from build123d import *

# Parameters (mm, degrees)
SKETCH1_R           = 1.8
BOSS_EXTRUDE1_DEPTH = 2
SKETCH2_W           = 12
SKETCH2_H           = 2
BOSS_EXTRUDE2_DEPTH = 20
SKETCH3_R           = 1.8
CUT_EXTRUDE1_DEPTH  = 56.195108479
BOSS_EXTRUDE3_DEPTH = 2
BOSS_EXTRUDE4_DEPTH = 2
FILLET1_R           = 5
FILLET2_R           = 5
FILLET3_R           = 1
FILLET4_R           = 1


with BuildPart() as part:
    # Sketch1 → Boss-Extrude1 (new body)
    with BuildSketch(Plane(origin=(0, 0, 0), x_dir=(1, 0, 0), z_dir=(0, 1, 0))):
        Polygon((-12.5, 19.5), (47.5, 19.5), (47.5, 9.5), (35, 9.5), (35, 0), (23, 0), (23, 9.5), (12, 9.5), (12, 0), (0, 0), (0, 9.5), (-12.5, 9.5), align=None)
        with Locations(Location((-7.5, 14.5, 0), (0, 0, 270))):
            Circle(SKETCH1_R, mode=Mode.SUBTRACT)
        with Locations(Location((42.5, 14.5, 0), (0, 0, 270))):
            Circle(SKETCH1_R, mode=Mode.SUBTRACT)
    extrude(amount=BOSS_EXTRUDE1_DEPTH)

    # Sketch2 → Boss-Extrude2 (add)
    with BuildSketch(Plane(origin=(0, 2, 0), x_dir=(1, 0, 0), z_dir=(0, 1, 0))):
        with Locations((29, 1)):
            Rectangle(SKETCH2_W, SKETCH2_H)
        with Locations((6, 1)):
            Rectangle(SKETCH2_W, SKETCH2_H)
    extrude(amount=BOSS_EXTRUDE2_DEPTH)

    # Sketch3 → Cut-Extrude1 (cut, through all)
    with BuildSketch(Plane(origin=(0, 0, -2), x_dir=(-1, 0, 0), z_dir=(0, 0, -1))):
        with Locations((-7, 7)):
            Circle(SKETCH3_R)
        with Locations((-7, 17)):
            Circle(SKETCH3_R)
        with Locations((-28, 7)):
            Circle(SKETCH3_R)
        with Locations((-28, 17)):
            Circle(SKETCH3_R)
    extrude(amount=-CUT_EXTRUDE1_DEPTH, mode=Mode.SUBTRACT)

    # Sketch4 → Boss-Extrude3 (add)
    with BuildSketch(Plane.ZY):
        Polygon((-2, 22), (-2, 2), (-19.5, 2), align=None)
    extrude(amount=-BOSS_EXTRUDE3_DEPTH)

    # Sketch5 → Boss-Extrude4 (add)
    with BuildSketch(Plane(origin=(35, 0, 0), x_dir=(0, 0, -1), z_dir=(1, 0, 0))):
        Polygon((2, 22), (2, 2), (19.5, 2), align=None)
    extrude(amount=-BOSS_EXTRUDE4_DEPTH)

    # Fillet1
    fillet1_edges = [part.edges().sort_by_distance(p)[0] for p in [
        (35, 1, -9.5),
        (23, 1, -9.5),
        (12, 1, -9.5),
        (0, 1, -9.5),
    ]]
    fillet(fillet1_edges, radius=FILLET1_R)

    # Fillet2
    fillet2_edges = [part.edges().sort_by_distance(p)[0] for p in [
        (47.5, 1, -9.5),
        (47.5, 1, -19.5),
        (-12.5, 1, -19.5),
        (-12.5, 1, -9.5),
    ]]
    fillet(fillet2_edges, radius=FILLET2_R - 0.0001)  # a hair under: the kernel refuses the full size

    # Fillet3
    fillet3_edges = [part.edges().sort_by_distance(p)[0] for p in [
        (33, 2, -10.75),
        (33, 12, -2),
        (35, 2, -12),
        (7, 2, -2),
        (2, 12, -2),
        (2, 2, -10.75),
        (0, 2, -12),
        (28, 2, -2),
    ]]
    fillet(fillet3_edges, radius=FILLET3_R)

    # Fillet4
    fillet4_edges = [part.edges().sort_by_distance(p)[0] for p in [
        (0, 22, -1),
        (12, 22, -1),
        (23, 22, -1),
        (35, 22, -1),
    ]]
    fillet(fillet4_edges, radius=FILLET4_R)


solid = part.part
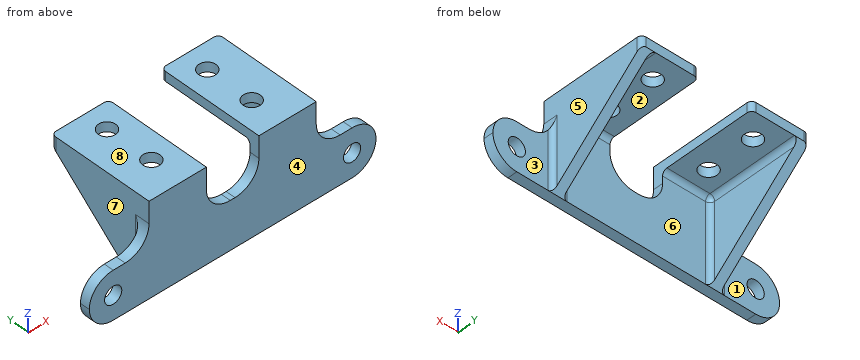
Input: part model. Units: mm. Frame: model coordinates. Face numbers are marked on the shaded views. A direction names the side the tool comes from. Give positions to 0.01 mm unless a question says otherwise; leave off trailing zeros. Loops run counter-clockwise (first coordinate to the right, second up) from the corner with the lowest first, then second, coordinate; pieces in that order, holes last. Notation, with made-up numbers: M -21,50.5 L 22,50.5 A14 cw 22,59.5 Z; hole C 9.25,-32.75 d5. An arc over 180 degrees is marked long. Use one line per item in the form item = value.
1. Reachability of the marked faces 1, 2, 3 and 4 from +Z, -Z, +X, -X, +Y, -Y: full face, straight path, thin tool, end or side. Return the list, or none.
Numbers:
face_1 = +Z, -Z, -X, +Y
face_2 = -Z, +Y
face_3 = +Z, -Z, +X, +Y
face_4 = +Z, -Z, +X, -X, -Y
2. First-contact query: pin 1 (3.5 mm diameter, centred on y = 5.5, z = -2.5, fed in from +X); pin 2 (9 mm diameter, centred on x = -4, z = -12, fed in from +Y); pin 3 (1.5 mm diameter, centred on y = 2.5, z = -11.5, fed in from -X). Flat tips, straight axial feed; report the tip coordinate or a pass-through.
Numbers:
pin_1 = 35
pin_2 = 12.93
pin_3 = -11.86
3. Section query D-D, the plane y = 3.75. Return the cut outline in (x, z).
Numbers:
outline = M 0,-17.97 L 2,-17.97 L 2,-3 A1 cw 3,-2 L 12,-2 L 12,0 L 0,0 Z; M 23,-2 L 32,-2 A1 cw 33,-3 L 33,-17.97 L 35,-17.97 L 35,0 L 23,0 Z
4. Section query C-C, the plane z = -8.75. Return the cut outline in (x, y), and give its area (3 significant figures).
Numbers:
outline = M -2.37,0 L 14.37,0 L 14.37,2 L 3,2 A1 cw 2,3 L 2,14.29 L 0,14.29 L 0,3 A1 cw -1,2 L -2.37,2 Z; M 20.63,0 L 37.37,0 L 37.37,2 L 36,2 A1 cw 35,3 L 35,14.29 L 33,14.29 L 33,3 A1 cw 32,2 L 20.63,2 Z
area = 117 mm²
5. Section query A-A, the plane x = 7. Return the cut outline in (y, z).
Numbers:
outline = M 0,-19.5 L 2,-19.5 L 2,-3 A1 cw 3,-2 L 5.2,-2 L 5.2,0 L 0,0 Z; M 8.8,-2 L 15.2,-2 L 15.2,0 L 8.8,0 Z; M 18.8,-2 L 22,-2 L 22,0 L 18.8,0 Z
6. Section query B-B, the plane y = 17. Return the cut outline in (x, z) (3 decimals).
Numbers:
outline = M 0,-6.375 L 2,-6.375 L 2,-3 A1 cw 3,-2 L 5.2,-2 L 5.2,0 L 0,0 Z; M 8.8,-2 L 12,-2 L 12,0 L 8.8,0 Z; M 23,-2 L 26.2,-2 L 26.2,0 L 23,0 Z; M 29.8,-2 L 32,-2 A1 cw 33,-3 L 33,-6.375 L 35,-6.375 L 35,0 L 29.8,0 Z
7. Line query: L1, parallel to Y at x = 7, z = -1.4; L2, parallel to X at y = 1.2, z = -14.5; L3, parallel to X at y = 9.25, z = -9.5. Output: solid intervals per line, ascending.
Numbers:
L1 = 0 to 5.2, 8.8 to 15.2, 18.8 to 22
L2 = -12.5 to -9.3, -5.7 to 40.7, 44.3 to 47.5
L3 = 0 to 2, 33 to 35
8. Pull-direction query (X, two-part tool) for the marked faces 5, 6, 7 and 8; classes: released by +X, released by -X, zero draft, split by the parting line, or undercut.
Numbers:
face_5 = released by +X
face_6 = undercut
face_7 = released by -X
face_8 = zero draft
